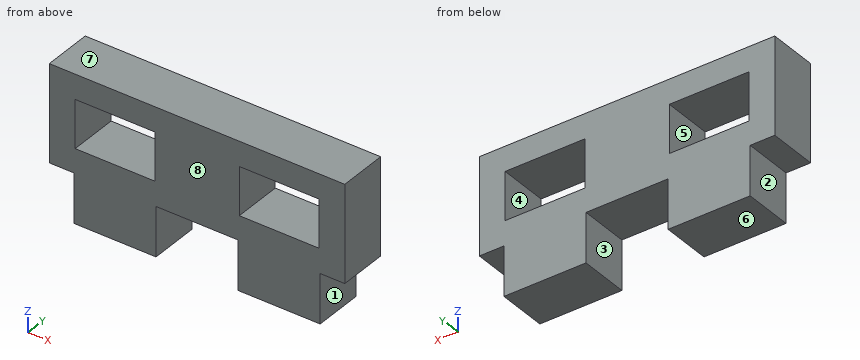
Autodesk Inventor part; units mm, degrees
ref_plane "YZ Plane" through (0, 0, 0) normal (1, 0, 0) x (0, 1, 0)
ref_plane "XZ Plane" through (0, 0, 0) normal (0, 1, 0) x (-1, 0, 0)
ref_plane "XY Plane" through (0, 0, 0) normal (0, 0, 1) x (1, 0, 0)
sketch "Sketch1" plane through (0, 0, 0) normal (0, 1, 0) x (-1, 0, 0)
  line L0 (-18, -5.8998) -> (-18, 5.8998)
  line L1 (-18, 5.8998) -> (18, 5.8998)
  line L2 (18, 5.8998) -> (18, -5.8998)
  line L3 (15, -11.8998) -> (5, -11.8998)
  line L4 (5, -11.8998) -> (5, -5.8998)
  line L5 (15, -5.8998) -> (15, -11.8998)
  line L6 (18, -5.8998) -> (15, -5.8998)
  line L7 (5, -5.8998) -> (-18, -5.8998) construction
  line L8 (-5, -11.8998) -> (-15, -11.8998)
  line L9 (-15, -11.8998) -> (-15, -5.8998)
  line L10 (-5, -5.8998) -> (-5, -11.8998)
  line L11 (5, -5.8998) -> (-5, -5.8998)
  line L12 (-15, -5.8998) -> (-18, -5.8998)
  line L13 (14.85, -2.9502) -> (5.15, -2.9502)
  line L14 (5.15, -2.9502) -> (5.15, 2.8998)
  line L15 (5.15, 2.8998) -> (14.85, 2.8998)
  line L16 (14.85, 2.8998) -> (14.85, -2.9502)
  line L17 (-5.15, 2.8998) -> (-5.15, -2.9502)
  line L18 (-5.15, -2.9502) -> (-14.85, -2.9502)
  line L19 (-14.85, -2.9502) -> (-14.85, 2.8998)
  line L20 (-14.85, 2.8998) -> (-5.15, 2.8998)
  line L21 (5.15, 2.8998) -> (-5.15, 2.8998) construction
  point P0 (0, 0)
  point P1 (18, 0)
  point P2 (0, -5.8998)
  point P3 (0, 5.8998)
  point P4 (0, 2.8998)
  dimension "d9" = 10
  dimension "d11" = 6
  dimension "d12" = 3
  dimension "d38" = 20
  dimension "d51" = 3
  dimension "d54" = 9.7
  dimension "d55" = 5.85
  dimension "d58" = 20
  dimension "d64" = 3
extrude "Extrusion1" add sketch "Sketch1" along normal blind 6
equation "\"d9\" = fingerW"
equation "\"d11\" = fingerH"
equation "\"d38\" = fingerSpacing"
equation "\"d54\" = fingerholeW"
equation "\"d55\" = fingerholeH"
equation "\"d58\" = fingerSpacing"
equation "\"d65\" = thickness"
equation "\"moduleWidth\" = 118"
equation "\"moduleHeight\" = 96"
equation "\"moduleMountD\" = 6.8"
equation "\"moduleCornerR\" = 5"
equation "\"d4\" = moduleCornerR"
equation "\"d5\" = moduleMountD"
equation "\"d6\" = moduleMountD"
equation "\"d8\" = moduleMountD"
equation "\"d10\" = moduleMountD"
equation "\"moduleOpeningR\" = 25"
equation "\"d13\" = moduleOpeningR"
equation "\"thickness\" = 6"
equation "\"d15\" = thickness"
equation "\"d16\" = 0"
equation "\"kerf\" = 0.15"
equation "\"fingerW\" = 10"
equation "\"fingerSpacing\" = 20"
equation "\"fingerholeW\" = fingerW - 2 * kerf"
equation "\"fingerholeH\" = thickness - kerf"
equation "\"moduleMountClearance\" = 19"
equation "\"actuatorW\" = 28"
equation "\"actuatorH\" = 40.8"
equation "\"openingMFC\" = 45"
equation "\"d28\" = thickness"
equation "\"d29\" = thickness"
equation "\"d30\" = 0.5 * actuatorH + thickness"
equation "\"d32\" = fingerholeH"
equation "\"d33\" = fingerholeW"
equation "\"d41\" = fingerholeH"
equation "\"d42\" = fingerholeW"
equation "\"supportSpacingFromMounting\" = 15"
equation "\"d52\" = 58.075"
equation "\"d53\" = 9.475"
equation "\"d0\" = moduleHeight"
equation "\"d1\" = moduleWidth"
equation "\"d17\" = openingMFC"
equation "\"d19\" = moduleMountClearance"
equation "\"d31\" = 15"
equation "\"supportXW\" = -2 * thickness + moduleMountW - 2 * supportSpacingFromMounting + kerf"
equation "\"chairThickness\" = 12.7"
equation "\"supportL\" = -chairThickness + dildoL + actuatorMountL - thickness"
equation "\"fingerH\" = thickness"
equation "\"d18\" = fingerH"
equation "\"d24\" = supportL"
equation "\"d44\" = thickness"
equation "\"d47\" = 0"
properties part number "6mm-Laser-Kerf-Test"
The listing builds one solid part. Answer for the finished solid, in the listing's coordinates (mm). Face numbers are marked on the shaded views. A direction names the side the tool comes from. Give positions to 0.01 mm unless a question says otherwise; leave off trailing zeros. Order: outer loops, then holes, each group sorted by start corner. A loop starts at its lowest first (then second) coordinate and runs counter-clockwise, first axis right, second up. Notation, with made-up numbers: (45, -39.5) - (73, -39.5) arc R30 cw to (73, -14.5) - close; hole circle Ø9 at (-39, -26). An arc over 180 degrees is marked (long way). One line per item, written item: value. Start each with the question number.
1) The mould has two halves that part along Z. Classify the marked faces 5, 6, 7 and 8: released by +Z, released by -Z, zero draft, split by the parting line, or undercut.
2) Given pin 1 Ø3 at (y, z) = (4.5, -10.5) entering from -X; pin 2 Ø3.5 at (x, y) = (17, 3.5) entering from -Z; pin 3 Ø1.8 at (y, z) = (3, -8) entering from +X; pin 4 Ø6 at (x, z) = (10, -4.5) entering from -Y, each flat-ended and moving along its own axis, determine where each tip first touches the part or whether it passes through.
3) A cutting plane is placed at D-D on z = -10.25. Give the vertices of the cut face in (x, y), then the cut area to 3 significant figures.
4) Find the intervals of material crossed by L1, parallel to X at y = 2.35, z = 2.5; L2, parallel to Z at x = 9, y = 2.8; L3, parallel to X at y = 1.3, z = -8.5, in increasing order.
5) A tool of negligible diameter and unlimited length cuts with its end or side. For the marked faces 1, 2, 3 and 4, from which of +Z, -Z, +X, -X, +Y, -Y can it reach the whole face along a straight path? Write none if from no direction.
6) A cutting plane is placed at A-A on z = 2.25. Give the vertices of the cut face in (x, y).
7) A cutting plane is placed at B-B on x = 12. Give the vertices of the cut face in (y, z), then the cut area to 3 significant figures.
8) A cutting plane is placed at C-C on y = 2. Give the vertices of the cut face in (x, z), then the cut area to 3 significant figures.
Answer sheet:
1. face 5: undercut
1. face 6: released by -Z
1. face 7: released by +Z
1. face 8: zero draft
2. pin 1: stops at x = -15
2. pin 2: stops at z = -5.9
2. pin 3: stops at x = 15
2. pin 4: stops at y = 0
3. outline: (-15, 0) - (-5, 0) - (-5, 6) - (-15, 6) - close; (5, 0) - (15, 0) - (15, 6) - (5, 6) - close
3. area: 120 mm2
4. L1: x = -18 to -14.85, -5.15 to 5.15, 14.85 to 18
4. L2: z = -11.9 to -2.95, 2.9 to 5.9
4. L3: x = -15 to -5, 5 to 15
5. face 1: -Z, +X, +Y, -Y
5. face 2: -Z, -X, +Y, -Y
5. face 3: -Z, +Y, -Y
5. face 4: +Y, -Y
6. outline: (-18, 0) - (-14.85, 0) - (-14.85, 6) - (-18, 6) - close; (-5.15, 0) - (5.15, 0) - (5.15, 6) - (-5.15, 6) - close; (14.85, 0) - (18, 0) - (18, 6) - (14.85, 6) - close
7. outline: (0, -11.9) - (6, -11.9) - (6, -2.95) - (0, -2.95) - close; (0, 2.9) - (6, 2.9) - (6, 5.9) - (0, 5.9) - close
7. area: 71.7 mm2
8. outline: (-18, -5.9) - (-15, -5.9) - (-15, -11.9) - (-5, -11.9) - (-5, -5.9) - (5, -5.9) - (5, -11.9) - (15, -11.9) - (15, -5.9) - (18, -5.9) - (18, 5.9) - (-18, 5.9) - close; hole (-14.85, -2.95) - (-5.15, -2.95) - (-5.15, 2.9) - (-14.85, 2.9) - close; hole (5.15, -2.95) - (14.85, -2.95) - (14.85, 2.9) - (5.15, 2.9) - close
8. area: 431 mm2
